from build123d import *

# Parameters (mm, degrees)
SKETCH1_W           = 340
SKETCH1_H           = 54
BOSS_EXTRUDE1_DEPTH = 120
SHELL1_T            = 2.5
SKETCH2_R           = 52.5
CUT_EXTRUDE1_DEPTH  = 10
SKETCH3_W           = 300
SKETCH3_H           = 40
CUT_EXTRUDE2_DEPTH  = 10
SKETCH4_W           = 100
SKETCH4_H           = 25
CUT_EXTRUDE3_DEPTH  = 341
SKETCH5_W           = 40
SKETCH5_H           = 90
CUT_EXTRUDE4_DEPTH  = 10
SKETCH6_W           = 330
SKETCH6_H           = 10
CUT_EXTRUDE5_DEPTH  = 10


with BuildPart() as part:
    # Sketch1 → Boss-Extrude1 (new body)
    with BuildSketch(Plane.XY):
        Rectangle(SKETCH1_W, SKETCH1_H)
    extrude(amount=BOSS_EXTRUDE1_DEPTH)

    # Shell1 (no face opened: a closed hollow body)
    add(offset(amount=-SHELL1_T, mode=Mode.PRIVATE), mode=Mode.SUBTRACT)

    # Sketch2 → Cut-Extrude1 (cut)
    with BuildSketch(Plane(origin=(0, 27, 0), x_dir=(1, 0, 0), z_dir=(0, 1, 0))):
        with Locations((-110, -60)):
            Circle(SKETCH2_R)
        with Locations((0, -60)):
            Circle(SKETCH2_R)
        with Locations((110, -60)):
            Circle(SKETCH2_R)
    extrude(amount=-CUT_EXTRUDE1_DEPTH, mode=Mode.SUBTRACT)

    # Sketch3 → Cut-Extrude2 (cut)
    with BuildSketch(Plane.XY.offset(120)):
        Rectangle(SKETCH3_W, SKETCH3_H)
    extrude(amount=-CUT_EXTRUDE2_DEPTH, mode=Mode.SUBTRACT)

    # Sketch4 → Cut-Extrude3 (cut, through all)
    with BuildSketch(Plane(origin=(170, 0, 0), x_dir=(0, 0, -1), z_dir=(1, 0, 0))):
        with Locations((-60, -12)):
            Rectangle(SKETCH4_W, SKETCH4_H)
    extrude(amount=-CUT_EXTRUDE3_DEPTH, mode=Mode.SUBTRACT)

    # Sketch5 → Cut-Extrude4 (cut)
    with BuildSketch(Plane.XZ.offset(27)):
        with Locations((140, 58.55655344)):
            Rectangle(SKETCH5_W, SKETCH5_H)
    extrude(amount=-CUT_EXTRUDE4_DEPTH, mode=Mode.SUBTRACT)

    # Sketch6 → Cut-Extrude5 (cut)
    with BuildSketch(Plane(origin=(0, 0, 0), x_dir=(-1, 0, 0), z_dir=(0, 0, -1))):
        with Locations((0, -19.5)):
            Rectangle(SKETCH6_W, SKETCH6_H)
    extrude(amount=-CUT_EXTRUDE5_DEPTH, mode=Mode.SUBTRACT)


solid = part.part
Read the model definition and answer for the solid it produces. Units are mm, in the model's axes. A direction names the side the tool comes from. Give positions to 0.01 mm unless a question says otherwise; leave off trailing zeros. Write each loop counter-clockwise with the first axis right and the second up, starting at its lowest first coordinate (ties: lowest second). Pieces come first, ordered by that corner, then holes. Notation, with made-up numbers: (-2, -14) - (52, -14) arc R35 ccw to (52, 20) - close; hole circle Ø10 at (74.5, 4). An arc over 180 degrees is marked (long way). Return JSON: item names as keys, results as strings.
Q1. For a pull along Z with two mould halves and no side action, classify faces 4 (the face through (-2, -27, 59)), 5 (the face through (-1, 22, 120)), 6 (the face through (167.5, 11, 59)) as released by +Z, released by -Z, zero draft, split by the parting line, or undercut.
Reply:
{"face 4": "zero draft", "face 5": "released by +Z", "face 6": "undercut"}
Q2. For faces 1 (the face through (158.5, 25.8, 80.1)), 2 (the face through (-2, 6, 2.5)), 3 (the face through (-170, 12, 59)), determine the directions among +Z, -Z, +X, -X, +Y, -Y from which every point of the face is accessible in a straight line to the end or side of a thin tool.
Reply:
{"face 1": "+Y", "face 2": "none", "face 3": "+Z, -Z, -X, +Y, -Y"}
Q3. A cutting plane is placed at B-B, the plane y = -10. Determine the outline of the cut face in (x, z).
Reply:
{"outline": "(-170, 0) - (170, 0) - (170, 10) - (167.5, 10) - (167.5, 2.5) - (-167.5, 2.5) - (-167.5, 10) - (-170, 10) - close; (-170, 110) - (-167.5, 110) - (-167.5, 117.5) - (-150, 117.5) - (-150, 120) - (-170, 120) - close; (150, 117.5) - (167.5, 117.5) - (167.5, 110) - (170, 110) - (170, 120) - (150, 120) - close"}
Q4. Given P1, Ø4, axis at x = 124, y = 4, coming from the +Z side; P2, Ø8, axis at x = -100.5, y = 6, coming from the -Z side, each flat-ended and moving along its own axis, determine where each tip first touches the part or whether it passes through.
Reply:
{"P1": "z = 2.5", "P2": "z = 0"}
Q5. A cutting plane is placed at A-A, the plane x = 110. Determine the outline of the cut face in (y, z).
Reply:
{"outline": "(-27, 0) - (-24.5, 0) - (-24.5, 117.5) - (-20, 117.5) - (-20, 120) - (-27, 120) - close; (-14.5, 0) - (27, 0) - (27, 7.5) - (24.5, 7.5) - (24.5, 2.5) - (-14.5, 2.5) - close; (20, 117.5) - (24.5, 117.5) - (24.5, 112.5) - (27, 112.5) - (27, 120) - (20, 120) - close"}
Q6. A cutting plane is placed at D-D, the plane y = 6.5. Determine the outline of the cut face in (x, z), and give its area (4 significant figures).
Reply:
{"outline": "(-170, 0) - (170, 0) - (170, 120) - (150, 120) - (150, 117.5) - (167.5, 117.5) - (167.5, 2.5) - (-167.5, 2.5) - (-167.5, 117.5) - (-150, 117.5) - (-150, 120) - (-170, 120) - close", "area": "1,525 mm²"}
Q7. A cutting plane is placed at C-C, the plane z = 60. Determine the outline of the cut face in (x, y).
Reply:
{"outline": "(-170, -27) - (120, -27) - (120, -24.5) - (-170, -24.5) - close; (-170, 0.5) - (-167.5, 0.5) - (-167.5, 24.5) - (-162.5, 24.5) - (-162.5, 27) - (-170, 27) - close; (-57.5, 24.5) - (-52.5, 24.5) - (-52.5, 27) - (-57.5, 27) - close; (52.5, 24.5) - (57.5, 24.5) - (57.5, 27) - (52.5, 27) - close; (160, -27) - (170, -27) - (170, -24.5) - (160, -24.5) - close; (162.5, 24.5) - (167.5, 24.5) - (167.5, 0.5) - (170, 0.5) - (170, 27) - (162.5, 27) - close"}
Q8. Consider line 1 along X through (y, z) = (25.5, 60); line 2 along X through (y, z) = (-10, 9); line 3 along Y through (x, z) = (69, 18.5). Determine where each line is inside the solid, lowest interval first. Write a range as [from, to].
Reply:
{"line 1": "[-170, -162.5], [-57.5, -52.5], [52.5, 57.5], [162.5, 170]", "line 2": "[-170, -167.5], [167.5, 170]", "line 3": "[-27, -24.5], [24.5, 27]"}
